Geometry check sheet. Reference: the model listing, model coordinates, mm. Face numbers are marked on the shaded views. Give positions to 0.01 mm unless a question says otherwise; leave off trailing zeros. Loops run counter-clockwise (first coordinate to the right, second up) from the corner with the lowest first, then second, coordinate; pieces in that order, holes last.
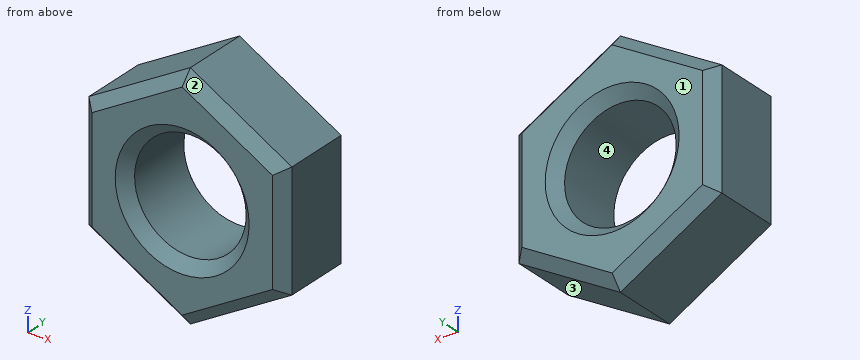
```python
from build123d import *

# Parameters (mm, degrees)
ESQUISSE1_R        = 1.5
BOSS_EXTRU_1_DEPTH = 2.4
CHANFREIN1_SIZE    = 0.3


with BuildPart() as part:
    # Esquisse1 → Boss.-Extru.1 (new body)
    with BuildSketch(Plane(origin=(0, 0, 0), x_dir=(1, 0, 0), z_dir=(0, 1, 0))):
        Polygon((0, 3.15), (-2.727980022, 1.575), (-2.727980022, -1.575), (0, -3.15), (2.727980022, -1.575), (2.727980022, 1.575), align=None)
        with Locations(Location((0, 0, 0), (0, 0, 270))):
            Circle(ESQUISSE1_R, mode=Mode.SUBTRACT)
    extrude(amount=BOSS_EXTRU_1_DEPTH)

    # Chanfrein1
    chanfrein1_edges = [part.edges().sort_by_distance(p)[0] for p in [
        (-2.727980022, 2.4, 0),
        (-1.363990011, 2.4, 2.3625),
        (0, 0, -1.5),
        (0, 2.4, -1.5),
        (1.363990011, 2.4, 2.3625),
        (2.727980022, 2.4, 0),
        (1.363990011, 2.4, -2.3625),
        (2.727980022, 0, 0),
        (1.363990011, 0, 2.3625),
        (-1.363990011, 0, 2.3625),
        (-2.727980022, 0, 0),
        (-1.363990011, 0, -2.3625),
        (1.363990011, 0, -2.3625),
        (-1.363990011, 2.4, -2.3625),
    ]]
    chamfer(chanfrein1_edges, length=CHANFREIN1_SIZE)


solid = part.part
```
1) Mould release check, pull along Z, two halves, no side actions. Record for the marked faces 1, 2, 3 and 4: +Z half, -Z half, draft (parallel to the pull), parting line (faces both ways), or undercut.
2) Depth check by flat-ended pin: P1, Ø1.8, axis at x = 0, z = 0, coming from the +Y side. Enter the tip coordinate at first touch or a pass-through.
3) Sectioned sample at A-A on z = 0. Enter the section's corners in (x, y).
4) Sectioned sample at D-D on x = -1.9. Enter the section's corners in (y, z), plus the area to 3 significant figures.
5) Sectioned sample at C-C on x = 2.3. Enter the section's corners in (y, z), plus the area to 3 significant figures.
6) Sectioned sample at B-B on y = 1. Enter the section's corners in (x, z) (3 decimals), plus the area to 3 significant figures.
7) Scan lines: line 1 along X through (y, z) = (1.3, 0); line 2 along X through (y, z) = (1.6, -0.5); line 3 along Z through (x, y) = (-0.25, 1.75). Record each from-to range of solid material in increasing order.
Determined:
1. face 1: draft
1. face 2: +Z half
1. face 3: -Z half
1. face 4: undercut
2. P1: passes through
3. outline: (-2.73, 0.3) - (-2.43, 0) - (-1.8, 0) - (-1.5, 0.3) - (-1.5, 2.1) - (-1.8, 2.4) - (-2.43, 2.4) - (-2.73, 2.1) - close; (1.5, 0.3) - (1.8, 0) - (2.43, 0) - (2.73, 0.3) - (2.73, 2.1) - (2.43, 2.4) - (1.8, 2.4) - (1.5, 2.1) - close
4. outline: (0, -1.71) - (0.3, -2.05) - (2.1, -2.05) - (2.4, -1.71) - (2.4, 1.71) - (2.1, 2.05) - (0.3, 2.05) - (0, 1.71) - close
4. area: 9.65 mm2
5. outline: (0, -1.48) - (0.3, -1.82) - (2.1, -1.82) - (2.4, -1.48) - (2.4, 1.48) - (2.1, 1.82) - (0.3, 1.82) - (0, 1.48) - close
5. area: 8.54 mm2
6. outline: (-2.728, -1.575) - (0, -3.15) - (2.728, -1.575) - (2.728, 1.575) - (0, 3.15) - (-2.728, 1.575) - close; hole circle Ø3 at (0, 0)
6. area: 18.7 mm2
7. line 1: x = -2.73 to -1.5, 1.5 to 2.73
7. line 2: x = -2.73 to -1.41, 1.41 to 2.73
7. line 3: z = -3.01 to -1.48, 1.48 to 3.01
